Can you work these out from the model? Positions are in its coordinate system, mm. Face numbers are marked on the shaded views. A direction names the side the tool comes from. Coordinates: 2 decimals unless noted, no trailing zeros. Write each loop counter-clockwise with the first axis right and the second up, starting at its lowest first coordinate (ties: lowest second). Pieces come first, ordered by that corner, then holes. Notation, with made-up numbers: (68.25, 64) -> (90.25, 64) arc R29 ccw to (90.25, 97) -> close; hole circle Ø2 at (-26.75, 69). An arc over 180 degrees is marked (long way). Use one line per item in the form item = value.
```python
from build123d import *

# Parameters (mm, degrees)
F0_W     = 12.5
F0_H     = 9
F1_DEPTH = 8
F2_R     = 2.15
F3_DEPTH = 6.5
F4_R     = 2


with BuildPart() as f1:
    # F0 (on Top) → F1 (new body)
    with BuildSketch(Plane.XY):
        Rectangle(F0_W, F0_H)
        with BuildLine():
            ThreePointArc((14.872505, 0), (11.113065, 3.307334), (6.25, 4.5))
            Line((6.25, 4.5), (6.25, -4.5))
            ThreePointArc((6.25, -4.5), (10.167104, -5.392854), (13.310355, -7.895026))
            Line((13.310355, -7.895026), (17.232623, -12.801666))
            ThreePointArc((17.232623, -12.801666), (24.927557, -18.927186), (34.516945, -21.112965))
            Line((34.516945, -21.112965), (123.75, -21.112965))
            Line((123.75, -21.112965), (123.75, -14.964157))
            Line((123.75, -14.964157), (33.715505, -14.964157))
            ThreePointArc((33.715505, -14.964157), (26.258617, -13.135356), (20.493996, -8.063982))
            Line((20.493996, -8.063982), (14.872505, 0))
        make_face()
    extrude(amount=F1_DEPTH)

    # F2 (on face) → F3 (cut)
    with BuildSketch(Plane(origin=(-6.25, 0, 0), x_dir=(0, -1, 0), z_dir=(-1, 0, 0))):
        with Locations((0, 4)):
            Circle(F2_R)
    extrude(amount=-F3_DEPTH, mode=Mode.SUBTRACT)

    # F4
    f4_edges = [f1.edges().sort_by_distance(p)[0] for p in [
        (-6.25, -4.5, 4),
        (123.75, -21.112965, 4),
        (123.75, -14.964157, 4),
        (-6.25, 4.5, 4),
    ]]
    fillet(f4_edges, radius=F4_R)


solid = f1.part
```
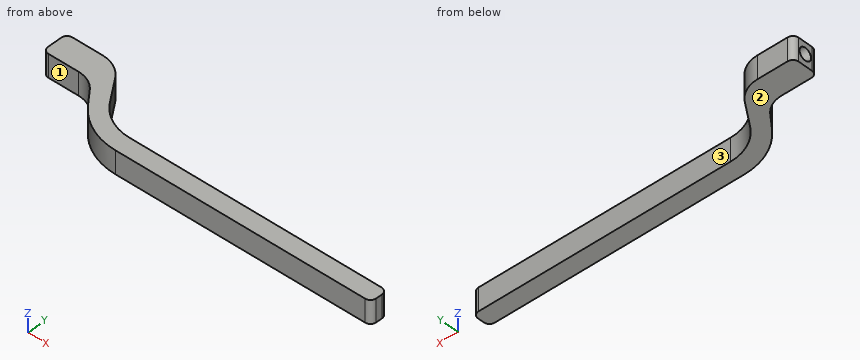
Q1. Suppose I cut it at A-A (z = 4). Write out the boundary of the cut face in (x, y).
Return value:
outline = (-6.25, -2.5) arc R2 ccw to (-4.25, -4.5) -> (6.25, -4.5) arc R9.04 cw to (13.31, -7.9) -> (17.23, -12.8) arc R22.13 ccw to (34.52, -21.11) -> (121.75, -21.11) arc R2 ccw to (123.75, -19.11) -> (123.75, -16.96) arc R2 ccw to (121.75, -14.96) -> (33.72, -14.96) arc R16.12 cw to (20.49, -8.06) -> (14.87, 0) arc R10.51 ccw to (6.25, 4.5) -> (-4.25, 4.5) arc R2 ccw to (-6.25, 2.5) -> (-6.25, 2.15) -> (0.25, 2.15) -> (0.25, -2.15) -> (-6.25, -2.15) -> close
Q2. Suppose I cut it at C-C (y = -10.5). Write out the boundary of the cut face in (x, z), then the cut area to 3 significant figures.
Return value:
outline = (15.39, 0) -> (22.58, 0) -> (22.58, 8) -> (15.39, 8) -> close
area = 57.5 mm2
Q3. If I drill on line 1 (Z direction, x = -3, y = 0); line 2 (Y direction, x = 110.5, z = 1.5); line 3 (X direction, y = -9, z = 1.5), over which ranges is the centre line in solid material (lowest first)? Write a range as from..to.
Return value:
line_1 = 0..1.85, 6.15..8
line_2 = -21.11..-14.96
line_3 = 14.19..21.2
Q4. Will these pins go through, and if not, where does the flat tip stop? pin 1 (2.5 mm diameter, centred on x = 69, z = 5.5, fed in from +Y); pin 2 (2.5 mm diameter, centred on y = 0, z = 4, fed in from -X); pin 3 (1.5 mm diameter, centred on y = -7, z = 1, fed in from -X).
Return value:
pin_1 = -14.96
pin_2 = 0.25
pin_3 = 11.6
Q5. Suppose I cut it at B-B (x = 100). Write out the boundary of the cut face in (y, z).
Return value:
outline = (-21.11, 0) -> (-14.96, 0) -> (-14.96, 8) -> (-21.11, 8) -> close
Q6. For the marked faces 1, 2 and 3, which set-ups out of +Z, -Z, +X, -X, +Y, -Y let a thin tool reach every point of the face, with its end or its side?
Return value:
face_1 = +Z, -Z, -X, -Y
face_2 = -Z, +X, -X, +Y, -Y
face_3 = +Z, -Z, +X, +Y
